```python
from build123d import *

# Parameters (mm, degrees)
SKETCH_2_R      = 2.75
EXTRUDE_1_DEPTH = 3
SKETCH_3_R      = 1.5
EXTRUDE_2_DEPTH = 35
FILLET_1_R      = 0.5


with BuildPart() as part:
    # ｽｹｯﾁ2 → ﾎﾞｽ - 押し出し1 (new body)
    with BuildSketch(Plane.XY):
        Circle(SKETCH_2_R)
    extrude(amount=EXTRUDE_1_DEPTH)

    # ｽｹｯﾁ3 → ﾎﾞｽ - 押し出し2 (add)
    with BuildSketch(Plane.XY.offset(3)):
        Circle(SKETCH_3_R)
    extrude(amount=EXTRUDE_2_DEPTH)

    # ﾌｨﾚｯﾄ1
    fillet_1_edges = [part.edges().sort_by_distance(p)[0] for p in [
        (-2.75, 0, 0),
    ]]
    fillet(fillet_1_edges, radius=FILLET_1_R)


solid = part.part
```
Geometry: final body of the model. Coordinates: model frame, mm. A direction names the side the tool comes from. Round coordinates to 2 decimals unless told otherwise and drop trailing zeros. Order: outer loops, then holes, each group sorted by start corner. A loop starts at its lowest first (then second) coordinate and runs counter-clockwise, first axis right, second up. Notation, with made-up numbers: (-1.5, 29.25) - (40.5, 29.25) arc R15 ccw to (40.5, 52.25) - close; hole circle Ø2 at (-18, 54). An arc over 180 degrees is marked (long way). Use CSV: the item, a comma, the result in double quotes. Start each with the question number.
Q1. Section query C-C (z = 10.5). Return loops of the section in (x, y), and give its area (3 significant figures).
Q2. Section query A-A (x = 0). Return loops of the section in (y, z), and give its area (3 significant figures).
Q3. Material intervals for line 1 along Z through (x, y) = (-1.45, -0.6); line 2 along Y through (x, z) = (0, 24.5); line 3 along X through (y, z) = (1.3, 6), sorted ascending. Write a range as from..to.
Q4. First-contact query: pin 1 (1 mm diameter, centred on x = 0, z = 30, fed in from +Y); pin 2 (2 mm diameter, centred on x = 1.5, z = 33.5, fed in from +Y). Flat tips, straight axial feed; report the tip coordinate or a pass-through.
Q5. Access query for faces 1 (the face through (-1.5, 0.07, 20.26)), 2 (the face through (-0.596, -2.685, 1.732)). Directions: +Z, -Z, +X, -X, +Y, -Y. A direction counts if a zero-diameter tool reaches every point of the face in a straight line with its end or side. Return the directions, or none.
Result set:
1,outline,"circle Ø3 at (0, 0)"
1,area,"7.07 mm2"
2,outline,"(-2.75, 0.5) arc R0.5 ccw to (-2.25, 0) - (2.25, 0) arc R0.5 ccw to (2.75, 0.5) - (2.75, 3) - (1.5, 3) - (1.5, 38) - (-1.5, 38) - (-1.5, 3) - (-2.75, 3) - close"
2,area,"121 mm2"
3,line 1,"z = 0..3"
3,line 2,"y = -1.5..1.5"
3,line 3,"x = -0.75..0.75"
4,pin 1,"stops at y = 1.5"
4,pin 2,"stops at y = 1.41"
5,face 1,"+Z"
5,face 2,"+Z, -Z"
